Study the drawing (mm; zero at the part's minimum x, y, z) and answer. A direction names the side the tool comes from. Give positions to 0.01 mm unless a question says otherwise; leave off trailing zeros. Order: outer loops, then holes, each group sorted by start corner. A loop starts at its lowest first (then second) coordinate and runs counter-clockwise, first axis right, second up.
Item 1: A cutting plane is placed at B-B (x = 7.5). Write down the section's boundary in (y, z), plus the area to 3 significant figures.
Item 2: A cutting plane is placed at A-A (z = 2.5). Write down the section's boundary in (x, y).
Item 3: The mould has two halves that part along Y. Classify the marked faces 1, 2, 3 and 4: +Y half, -Y half, draft (parallel to the pull), parting line (faces both ways), or undercut.
Item 4: Find the intervals of material crossed by line 1 along Y through (x, z) = (9.75, 4.3); line 2 along Z through (x, y) = (10.25, 2.75), in increasing order.
Item 5: A cutting plane is placed at C-C (y = 3). Write down the section's boundary in (x, z).
Item 6: Which of the six approach directions +Z, -Z, +X, -X, +Y, -Y give full straight-line access (tool end or side, diameter ignored) to the marked faces 5 and 6?
Item 7: Given pin 1 Ø0.5 at (x, y) = (5.5, 3) entering from +Z, flat-ended and moving along its own axis, determine where the tip first touches the part or whether it passes through.
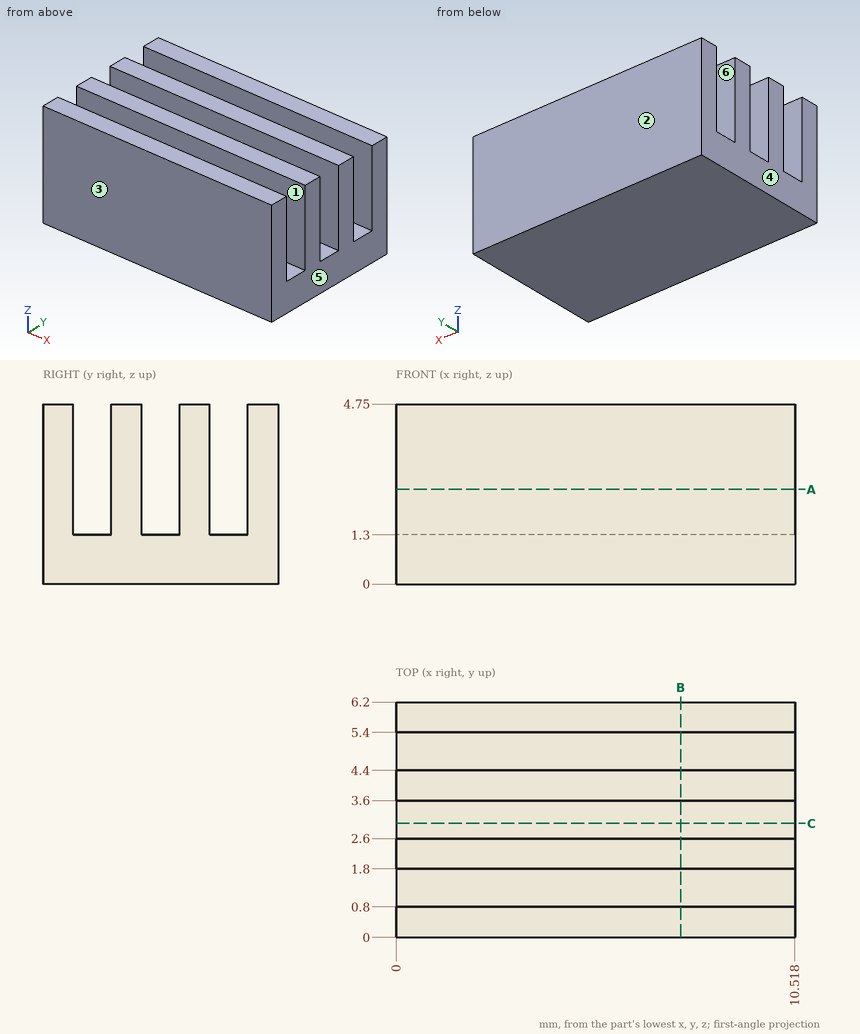
Response values:
1. outline: (0, 0) - (6.2, 0) - (6.2, 4.75) - (5.4, 4.75) - (5.4, 1.3) - (4.4, 1.3) - (4.4, 4.75) - (3.6, 4.75) - (3.6, 1.3) - (2.6, 1.3) - (2.6, 4.75) - (1.8, 4.75) - (1.8, 1.3) - (0.8, 1.3) - (0.8, 4.75) - (0, 4.75) - close
1. area: 19.1 mm2
2. outline: (0, 0) - (10.52, 0) - (10.52, 0.8) - (0, 0.8) - close; (0, 1.8) - (10.52, 1.8) - (10.52, 2.6) - (0, 2.6) - close; (0, 3.6) - (10.52, 3.6) - (10.52, 4.4) - (0, 4.4) - close; (0, 5.4) - (10.52, 5.4) - (10.52, 6.2) - (0, 6.2) - close
3. face 1: undercut
3. face 2: +Y half
3. face 3: -Y half
3. face 4: draft
4. line 1: y = 0 to 0.8, 1.8 to 2.6, 3.6 to 4.4, 5.4 to 6.2
4. line 2: z = 0 to 1.3
5. outline: (0, 0) - (10.52, 0) - (10.52, 1.3) - (0, 1.3) - close
6. face 5: +Z, -Z, +X, +Y, -Y
6. face 6: +Z, +X, -X
7. pin 1: stops at z = 1.3
